Part model, mm, in its own coordinate system. Face numbers are marked on the shaded views. A direction names the side the tool comes from. Round coordinates to 2 decimals unless told otherwise and drop trailing zeros. Loops run counter-clockwise (first coordinate to the right, second up) from the corner with the lowest first, then second, coordinate; pieces in that order, holes last. Notation, with made-up numbers: (5, 41) -> (39, 41) arc R16 cw to (39, 67) -> close; hole circle Ø10 at (41, 33.5). An arc over 180 degrees is marked (long way). Answer as CSV lines item,"result".
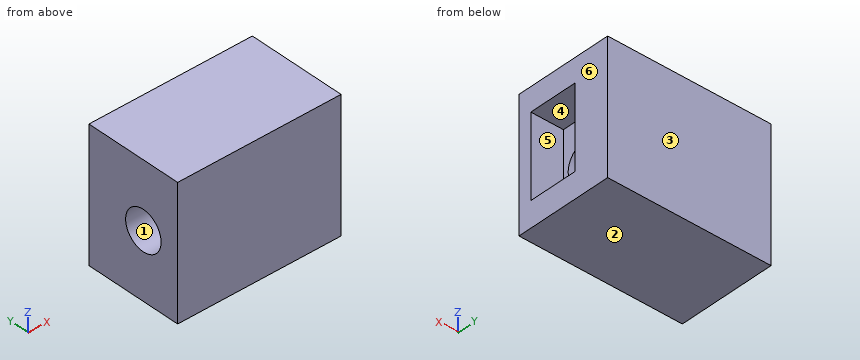
from build123d import *

# Parameters (mm, degrees)
F0_W      = 127.6799589396
F0_H      = 51.2897223234
F1_DEPTH  = 114.3676936626
F2_W      = 115.8702634275
F2_H      = 50.820171833
F3_DEPTH  = 25
F4_DEPTH  = 30
F7_W      = 250
F7_H      = 200
F8_DEPTH  = 150
F9_W      = 75
F9_H      = 125
F10_DEPTH = 50
F11_R     = 30
F12_DEPTH = 200.001


with BuildPart() as f1:
    # F0 (on Front) → F1 (new body)
    with BuildSketch(Plane.XZ):
        with Locations((63.8399794698, -56.7509904504)):
            Rectangle(F0_W, F0_H)
    extrude(amount=F1_DEPTH)


with BuildPart() as f3:
    # F2 (on Front) → F3 (new body)
    with BuildSketch(Plane.XZ):
        with Locations((103.8953531533, 116.1821186543)):
            Rectangle(F2_W, F2_H)
    extrude(amount=F3_DEPTH)

    # F4 (add): a face of the model
    f4_faces = [f3.faces().sort_by_distance(p)[0] for p in [
        (103.8953531533, -25, 116.1821186543),
    ]]
    extrude(f4_faces, amount=F4_DEPTH)


with BuildPart() as f8:
    # F7 (on Front) → F8 (new body)
    with BuildSketch(Plane.XZ):
        Rectangle(F7_W, F7_H)
    extrude(amount=F8_DEPTH)

    # F9 (on face) → F10 (cut)
    with BuildSketch(Plane.YZ.offset(125)):
        with Locations((-92.5, 1.5)):
            Rectangle(F9_W, F9_H)
    extrude(amount=-F10_DEPTH, mode=Mode.SUBTRACT)

    # F11 (on face) → F12 (cut, through all)
    with BuildSketch(Plane.YZ.offset(75)):
        with Locations((-92, 0)):
            Circle(F11_R)
    extrude(amount=-F12_DEPTH, mode=Mode.SUBTRACT)


solid = f8.part
Q1. Saw through at B-B, the plane x = 93.5. Write the cut outline in (y, z).
Geometry results:
outline,"(-150, -100) -> (0, -100) -> (0, 100) -> (-150, 100) -> close; hole (-130, -61) -> (-55, -61) -> (-55, 64) -> (-130, 64) -> close"
Q2. Saw through at A-A, the plane z = 0. Write the cut outline in (x, y), then the cut area to 4 significant figures.
Geometry results:
outline,"(-125, -150) -> (125, -150) -> (125, -130) -> (75, -130) -> (75, -122) -> (-125, -122) -> close; (-125, -62) -> (75, -62) -> (75, -55) -> (125, -55) -> (125, 0) -> (-125, 0) -> close"
area,"21,750 mm2"
Q3. Two-plate mould, pull along Y, no slides. Class the marked faces 1, 2, 3 and 4: pulls with the +Y half, pulls with the -Y half, needs draft (parallel to the pull), parting line crosses it, or undercut.
Geometry results:
face 1,"undercut"
face 2,"needs draft"
face 3,"pulls with the +Y half"
face 4,"undercut"
Q4. Drop a flat-ended pin along its axis: P1, Ø5, axis at y = -122.5, z = -45, coming from the +X side. Give the stop position or say it passes through.
Geometry results:
P1,"x = 75"
Q5. Saw through at C-C, the plane y = -92. Write the cut outline in (x, z).
Geometry results:
outline,"(-125, -100) -> (125, -100) -> (125, -61) -> (75, -61) -> (75, -30) -> (-125, -30) -> close; (-125, 30) -> (75, 30) -> (75, 64) -> (125, 64) -> (125, 100) -> (-125, 100) -> close"
Q6. Which spindle directions (+Z, -Z, +X, -X, +Y, -Y) get a long thin tool onto all of the face, cutting with end or side? Do the marked faces 5 and 6. Say none if no direction does.
Geometry results:
face 5,"+X"
face 6,"+Z, -Z, +X, +Y, -Y"
Q7. Drill centre lines: line 1 along Z through (x, y) = (91.5, -116.5); line 2 along Z through (x, y) = (11, -92); line 3 along Y through (x, z) = (-35.5, 11). Where is each one in solid material? Low to high.
Geometry results:
line 1,"-100 to -61, 64 to 100"
line 2,"-100 to -30, 30 to 100"
line 3,"-150 to -119.91, -64.09 to 0"
Q8. Saw through at D-D, the plane z = 36. Write the cut outline in (x, y), then the cut area to 4 significant figures.
Geometry results:
outline,"(-125, -150) -> (125, -150) -> (125, -130) -> (75, -130) -> (75, -55) -> (125, -55) -> (125, 0) -> (-125, 0) -> close"
area,"33,750 mm2"
